Part print with two shaded views. Sizes in mm from the minimum x, y, z corner. A direction names the side the tool comes from. Round coordinates to 2 decimals unless told otherwise and drop trailing zeros. Write each loop counter-clockwise with the first axis right and the second up, starting at its lowest first coordinate (ties: lowest second). Pieces come first, ordered by that corner, then holes. Notation, with made-up numbers: (5.5, 20.25) - (41.5, 20.25) arc R14 cw to (41.5, 26.25) - close; hole circle Ø10 at (-31, 4.25). An arc over 180 degrees is marked (long way). Use one line per item in the form item = value. Start each with the question number.
Item 1: Pull direction X, two halves, no side cores. Call the marked faces 6, 7, 8 and 9: +X half, -X half, draft (parallel to the pull), parting line (faces both ways), or undercut.
Item 2: Pin check, flat tips, straight feed: pin 1 (9.5 mm diameter, centred on x = 19, y = 52, fed in from -Z); pin 2 (16 mm diameter, centred on x = 22, z = 43.5, fed in from -Y); pin 3 (9.5 mm diameter, centred on x = 20.5, z = 52.5, fed in from +Y); pin 4 (10.5 mm diameter, centred on x = 16, y = 13, fed in from -Z). Stop position of each tip, or through.
Item 3: Drill centre lines: L1, parallel to Y at x = 16, z = 4.5; L2, parallel to Y at x = 3, z = 33; L3, parallel to Y at x = 14, z = 3.5. Where is each one in solid material? Low to high.
Item 4: Band-saw the part on A-A, the plane z = 25. List the corners of the cut face in (x, y), and give its area (3 significant figures).
Item 5: Band-saw the part on B-B, the plane y = 100. List the corners of the cut face in (x, z).
Item 6: Band-saw the part on D-D, the plane z = 40. List the corners of the cut face in (x, y).
Item 7: Tool access for the marked faces 1, 2, 3, 4 and 5: list every direction of +Z, -Z, +X, -X, +Y, -Y with a clear straight run to the whole face (end or side of a thin tool).
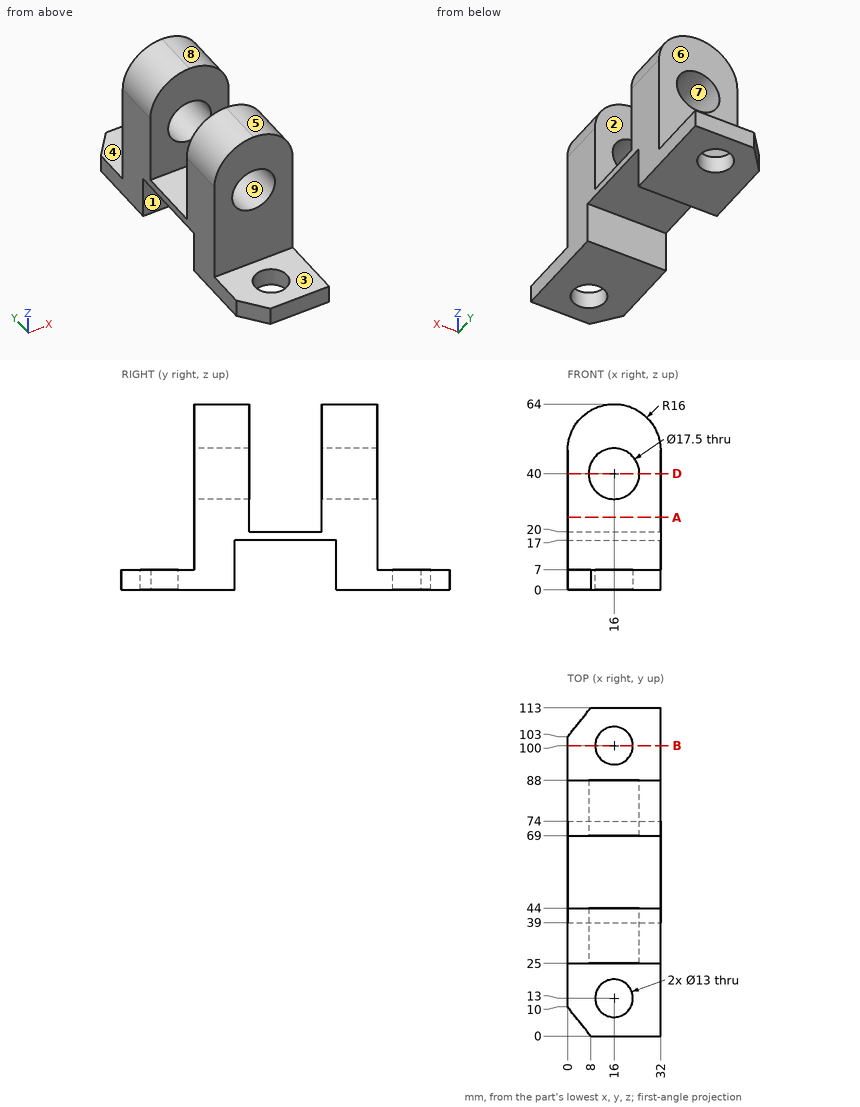
Determined:
q1.face_6 = draft
q1.face_7 = undercut
q1.face_8 = +X half
q1.face_9 = undercut
q2.pin_1 = 17
q2.pin_2 = 25
q2.pin_3 = 88
q2.pin_4 = through
q3.L1 = 0 to 6.5, 19.5 to 39, 74 to 93.5, 106.5 to 113
q3.L2 = 25 to 44, 69 to 88
q3.L3 = 0 to 6.82, 19.18 to 39, 74 to 93.82, 106.18 to 113
q4.outline = (0, 25) - (32, 25) - (32, 44) - (0, 44) - close; (0, 69) - (32, 69) - (32, 88) - (0, 88) - close
q4.area = 1,220 mm²
q5.outline = (0, 0) - (9.5, 0) - (9.5, 7) - (0, 7) - close; (22.5, 0) - (32, 0) - (32, 7) - (22.5, 7) - close
q6.outline = (0, 25) - (7.25, 25) - (7.25, 44) - (0, 44) - close; (0, 69) - (7.25, 69) - (7.25, 88) - (0, 88) - close; (24.75, 25) - (32, 25) - (32, 44) - (24.75, 44) - close; (24.75, 69) - (32, 69) - (32, 88) - (24.75, 88) - close
q7.face_1 = -Z, +X, -X
q7.face_2 = +Z, +X, -X
q7.face_3 = +Z, +X, -X, -Y
q7.face_4 = +Z, +X, -X, +Y
q7.face_5 = +Z, +X, +Y, -Y
